Can you work these out from the model? Positions are in its coordinate system, mm. A direction names the side the tool comes from. Give positions to 0.01 mm unless a question says otherwise; leave off trailing zeros. Order: outer loops, then holes, each group sorted by start corner. A loop starts at its lowest first (then second) coordinate and runs counter-clockwise, first axis right, second up.
```python
from build123d import *

# Parameters (mm, degrees)
SKETCH_1_R      = 2.5
SKETCH_1_R_2    = 0.75
EXTRUDE_1_DEPTH = 3
SKETCH_2_R      = 4
SKETCH_2_R_2    = 2.5
EXTRUDE_2_DEPTH = 2.5


with BuildPart() as part:
    # 草图1 → 凸台-拉伸1 (new, symmetric)
    with BuildSketch(Plane(origin=(0, 0, 0), x_dir=(1, 0, 0), z_dir=(0, 1, 0))):
        with Locations(Location((0, 0, 0), (0, 0, 270))):
            Circle(SKETCH_1_R)
        with Locations(Location((0, 0, 0), (0, 0, 270))):
            Circle(SKETCH_1_R_2, mode=Mode.SUBTRACT)
    extrude(amount=EXTRUDE_1_DEPTH, both=True)

    # 草图2 → 凸台-拉伸2 (add, symmetric)
    with BuildSketch(Plane(origin=(0, 0, 0), x_dir=(1, 0, 0), z_dir=(0, 1, 0))):
        with Locations(Location((0, 0, 0), (0, 0, 270))):
            Circle(SKETCH_2_R)
        with Locations(Location((0, 0, 0), (0, 0, 270))):
            Circle(SKETCH_2_R_2, mode=Mode.SUBTRACT)
    extrude(amount=EXTRUDE_2_DEPTH, both=True)


solid = part.part
```
1) If I drill on line 1 (X direction, y = -0.3, z = 0); line 2 (Y direction, x = -2, z = -3.25); line 3 (Z direction, x = -0.25, y = -0.7), over which ranges is the centre line in solid material (lowest first)?
2) Suppose I cut it at D-D (z = 1.75). Please give me the cut outline in (x, y), and give its area (3 significant figures).
3) Suppose I cut it at C-C (y = 1.75). Please give me the cut outline in (x, z), and give its area (3 significant figures).
4) I'm going to push flat-ended pins straight in: pin 1 Ø2 at (x, y) = (1.5, -2.5) entering from -Z; pin 2 Ø1.2 at (x, z) = (0, 0) entering from -Y. Where does each tip first touch, or does it pass through?
5) We'd pull the mould along X, two halves only. Please class faces 1 (the face through (2, -2.5, 2)), 2 (the face through (0.225, -0.042, 0.715)), 3 (the face through (-3.905, 0.035, -0.867)): +X half, -X half, draft (parallel to the pull), parting line (faces both ways), or undercut.
6) Suppose I cut it at B-B (z = 0). Please give me the cut outline in (x, y).
7) Which directions (+Z, -Z, +X, -X, +Y, -Y) give clear straight access to the entire face, cutting with the end or side of a thin tool? Please do faces 4 (the face through (-2.44, 2.75, -0.54)), 5 (the face through (-2.44, -2.75, -0.54)), 6 (the face through (1, -3, 1)).
8) Suppose I cut it at A-A (x = 0). Please give me the cut outline in (y, z), and give its area (3 significant figures).
Results:
1. line 1: x = -4 to -0.75, 0.75 to 4
1. line 2: y = -2.5 to 2.5
1. line 3: z = -3.99 to -0.71, 0.71 to 3.99
2. outline: (-3.6, -2.5) - (-1.79, -2.5) - (-1.79, -3) - (1.79, -3) - (1.79, -2.5) - (3.6, -2.5) - (3.6, 2.5) - (1.79, 2.5) - (1.79, 3) - (-1.79, 3) - (-1.79, 2.5) - (-3.6, 2.5) - close
2. area: 39.5 mm2
3. outline: circle Ø8 at (0, 0); hole circle Ø1.5 at (0, 0)
3. area: 48.5 mm2
4. pin 1: stops at z = -3.97
4. pin 2: passes through
5. face 1: draft
5. face 2: undercut
5. face 3: parting line
6. outline: (-4, -2.5) - (-2.5, -2.5) - (-2.5, -3) - (-0.75, -3) - (-0.75, 3) - (-2.5, 3) - (-2.5, 2.5) - (-4, 2.5) - close; (0.75, -3) - (2.5, -3) - (2.5, -2.5) - (4, -2.5) - (4, 2.5) - (2.5, 2.5) - (2.5, 3) - (0.75, 3) - close
7. face 4: +Y
7. face 5: -Y
7. face 6: +Z, -Z, +X, -X, -Y
8. outline: (-3, -2.5) - (-2.5, -2.5) - (-2.5, -4) - (2.5, -4) - (2.5, -2.5) - (3, -2.5) - (3, -0.75) - (-3, -0.75) - close; (-3, 0.75) - (3, 0.75) - (3, 2.5) - (2.5, 2.5) - (2.5, 4) - (-2.5, 4) - (-2.5, 2.5) - (-3, 2.5) - close
8. area: 36.0 mm2
